Input: part model. Units: mm. Frame: model coordinates. A direction names the side the tool comes from. Round coordinates to 2 decimals unless told otherwise and drop trailing zeros. Loops run counter-clockwise (first coordinate to the right, second up) from the corner with the lowest first, then second, coordinate; pieces in that order, holes last.
1) Ray query, line 1 along X through (y, z) = (74.5, 46.95); line 2 along Z through (x, y) = (170.5, 62); line 3 along Y through (x, z) = (138, 40). Return the intervals inside material, ascending.
2) Section D-D, the plane y = 39. Return loops of the section in (x, z), and give its area (3 significant figures).
3) Section B-B, the plane z = 24.5. Return loops of the section in (x, y).
4) Access query for faces 1 (the face through (201.525, 93, 12)), 2 (the face through (193, 88, 19.5)), 3 (the face through (173.241, 27, 28)), 4 (the face through (180.02, 74.49, 25.08)). Directions: +Z, -Z, +X, -X, +Y, -Y. A direction counts if a zero-diameter tool reaches every point of the face in a straight line with its end or side. Return the directions, or none.
5) Section C-C, the plane x = 63. Return loops of the section in (y, z), and give its area (3 significant figures).
6) Section A-A, the plane z = 41. State how many separate pieces and enclosed holes the cut face has, and give its area (3 significant figures).
7) First-contact query: pin 1 (13.5 mm diameter, centred on x = 112.5, z = 37, fed in from +Y); pin 2 (3 mm diameter, centred on x = 45, z = 9.5, fed in from -Y); pin 3 (12 mm diameter, centred on x = 70, z = 15, fed in from +Y); pin 4 (17.5 mm diameter, centred on x = 121.5, y = 35.5, fed in from +Z). Flat tips, straight axial feed; report the tip coordinate or a pass-through.
8) Draft query along Y for faces 5 (the face through (193, 88, 30.5)), 6 (the face through (48.241, 27, 28)), 7 (the face through (185.44, 94.15, 48.45)). Return one class per face: pulls with the +Y half, pulls with the -Y half, needs draft (parallel to the pull), parting line crosses it, or undercut.
from build123d import *

# Parameters (mm, degrees)
BOSS_EXTRUDE1_DEPTH              = 50
CUT_EXTRUDE1_REACH               = 346.227
CUT_EXTRUDE1_OFFSET_FROM_SURFACE = 10
SKETCH7_W                        = 40
SKETCH7_H                        = 243.120368846
CUT_EXTRUDE2_REACH               = 336.227
SKETCH8_W                        = 40
SKETCH8_H                        = 80.210678119
BOSS_EXTRUDE2_DEPTH              = 5
BOSS_EXTRUDE3_DEPTH              = 5
SKETCH12_W                       = 11
SKETCH12_H                       = 50
CUT_EXTRUDE3_DEPTH               = 20
SKETCH13_W                       = 50
SKETCH13_H                       = 57
BOSS_EXTRUDE4_DEPTH              = 218.275432638
CUT_EXTRUDE5_DEPTH               = 185.855610396
CUT_EXTRUDE5_DEPTH_BACK          = 0.48
SKETCH14_W                       = 40
SKETCH14_H                       = 43.7
SKETCH14_W_2                     = 1.85
CUT_EXTRUDE6_START               = -10
SKETCH15_W                       = 5.5
SKETCH15_H                       = 5
CUT_EXTRUDE6_DEPTH               = 10
SKETCH16_W                       = 125
SKETCH16_H                       = 35
CUT_EXTRUDE7_DEPTH               = 45
CUT_EXTRUDE8_DEPTH               = 5
CUT_EXTRUDE9_DEPTH               = 16.750003
CUT_EXTRUDE10_REACH              = 266.941
SKETCH19_W                       = 6.892135624
SKETCH19_H                       = 14.5
SKETCH20_R                       = 1.75
CUT_EXTRUDE11_DEPTH              = 5


with BuildPart() as part:
    # Sketch2 → Boss-Extrude1 (new body)
    with BuildSketch(Plane.XY):
        Polygon((218.275432638, 103.163478703), (218.275432638, 0), (0, 0), (0, 44.039493547), (0, 248.120368846), (173.241161391, 74.879207455), (201.525432638, 103.163478703), align=None)
    extrude(amount=BOSS_EXTRUDE1_DEPTH)

    # Cut-Extrude1: up to this face of the body (flat: up to its plane, moved by the offset)
    cut_extrude1_end = Plane(part.part.faces().sort_by_distance((86.620580695, 161.499788151, 25))[0]).offset(-CUT_EXTRUDE1_OFFSET_FROM_SURFACE)
    # Sketch7 → Cut-Extrude1 (cut, up to the picked face)
    with BuildSketch(Plane.ZY, mode=Mode.PRIVATE) as cut_extrude1_sk1:
        with Locations((25, 121.560184423)):
            Rectangle(SKETCH7_W, SKETCH7_H)
    cut_extrude1_tool1 = split(extrude(cut_extrude1_sk1.sketch, amount=-CUT_EXTRUDE1_REACH, mode=Mode.PRIVATE), bisect_by=cut_extrude1_end, keep=Keep.BOTH, mode=Mode.PRIVATE)
    add(cut_extrude1_tool1.solids().sort_by(Axis((0, 121.560184, 25), (1, 0, 0)))[0], mode=Mode.SUBTRACT)

    # Cut-Extrude2: up to this plane
    cut_extrude2_end = Plane(origin=(180.312229203, 67.808139643, 50), z_dir=(0.7071067811865477, -0.7071067811865474, 0))
    # Sketch8 → Cut-Extrude2 (cut, up to the surface)
    with BuildSketch(Plane(origin=(218.275432638, 0, 0), x_dir=(0, 0, -1), z_dir=(1, 0, 0)), mode=Mode.PRIVATE) as cut_extrude2_sk1:
        with Locations((-25, 55.808139644)):
            Rectangle(SKETCH8_W, SKETCH8_H)
    cut_extrude2_tool1 = split(extrude(cut_extrude2_sk1.sketch, amount=-CUT_EXTRUDE2_REACH, mode=Mode.PRIVATE), bisect_by=cut_extrude2_end, keep=Keep.BOTH, mode=Mode.PRIVATE)
    add(cut_extrude2_tool1.solids().sort_by_distance((218.275433, 55.80814, 25))[0], mode=Mode.SUBTRACT)

    # Sketch10 → Boss-Extrude2 (add)
    with BuildSketch(Plane.XY.offset(50)):
        Polygon((0, 248.120368846), (3.535533906, 251.655902752), (173.241161391, 81.950275267), (197.989898732, 106.699012609), (201.525432638, 103.163478703), (173.241161391, 74.879207455), align=None)
    extrude(amount=-BOSS_EXTRUDE2_DEPTH)

    # Sketch11 → Boss-Extrude3 (add)
    with BuildSketch(Plane(origin=(0, 0, 0), x_dir=(-1, 0, 0), z_dir=(0, 0, -1))):
        Polygon((-201.525432638, 103.163478703), (-197.989898732, 106.699012609), (-173.241161391, 81.950275267), (-3.535533906, 251.655902752), (0, 248.120368846), (-173.241161391, 74.879207455), align=None)
    extrude(amount=-BOSS_EXTRUDE3_DEPTH)

    # Sketch12 → Cut-Extrude3 (cut)
    with BuildSketch(Plane(origin=(49.180976968, -49.180976968, 0), x_dir=(0, 0, 1), z_dir=(-0.7071067811865435, 0.7071067811865517, 0))):
        with Locations((25, 213.447595361)):
            Rectangle(SKETCH12_W, SKETCH12_H)
    extrude(amount=-CUT_EXTRUDE3_DEPTH, mode=Mode.SUBTRACT)

    # Sketch13 → Boss-Extrude4 (add)
    with BuildSketch(Plane(origin=(218.275432638, 0, 0), x_dir=(0, 0, -1), z_dir=(1, 0, 0))):
        with Locations((-25, 28.5)):
            Rectangle(SKETCH13_W, SKETCH13_H)
    extrude(amount=-BOSS_EXTRUDE4_DEPTH)

    # Sketch14 → Cut-Extrude5 (cut, two sides: drawn at the far end of the back side and taken through both)
    with BuildSketch(Plane(origin=(124.060184423, 124.060184423, 0), x_dir=(0, 0, -1), z_dir=(0.7071067811865435, 0.7071067811865517, 0)).offset(-CUT_EXTRUDE5_DEPTH_BACK)):
        with Locations((-25, -47.702404639)):
            Rectangle(SKETCH14_W, SKETCH14_H)
        with Locations((-45.925, -47.702404639)):
            Rectangle(SKETCH14_W_2, SKETCH14_H)
        with Locations((-4.075, -47.702404639)):
            Rectangle(SKETCH14_W_2, SKETCH14_H)
    extrude(amount=CUT_EXTRUDE5_DEPTH + CUT_EXTRUDE5_DEPTH_BACK, mode=Mode.SUBTRACT)

    # Sketch15 → Cut-Extrude6 (cut)
    with BuildSketch(Plane(origin=(49.180976968, -49.180976968, 0), x_dir=(0, 0, 1), z_dir=(-0.7071067811865477, 0.7071067811865474, 0)).offset(CUT_EXTRUDE6_START)):
        with Locations((27.75, 177.467595361)):
            Rectangle(SKETCH15_W, SKETCH15_H)
        with Locations((22.25, 177.467595361)):
            Rectangle(SKETCH15_W, SKETCH15_H)
    extrude(amount=CUT_EXTRUDE6_DEPTH, mode=Mode.SUBTRACT)

    # Sketch16 → Cut-Extrude7 (cut)
    with BuildSketch(Plane.XY.offset(50)):
        with Locations((110.741161391, 27.5)):
            Rectangle(SKETCH16_W, SKETCH16_H)
    extrude(amount=-CUT_EXTRUDE7_DEPTH, mode=Mode.SUBTRACT)

    # Sketch17 → Cut-Extrude8 (cut)
    with BuildSketch(Plane.XY.offset(5)):
        with BuildLine():
            ThreePointArc((73.991161391, 27.5), (75.741161391, 25.75), (77.491161391, 27.5))
            Line((77.491161391, 27.5), (73.991161391, 27.5))
        make_face()
        with BuildLine():
            Line((73.991161391, 27.5), (77.491161391, 27.5))
            ThreePointArc((77.491161391, 27.5), (75.741161391, 29.25), (73.991161391, 27.5))
        make_face()
        with BuildLine():
            ThreePointArc((108.991161391, 27.5), (110.741161391, 25.75), (112.491161391, 27.5))
            Line((112.491161391, 27.5), (108.991161391, 27.5))
        make_face()
        with BuildLine():
            Line((108.991161391, 27.5), (112.491161391, 27.5))
            ThreePointArc((112.491161391, 27.5), (110.741161391, 29.25), (108.991161391, 27.5))
        make_face()
        with BuildLine():
            ThreePointArc((143.991161391, 27.5), (145.741161391, 25.75), (147.491161391, 27.5))
            Line((147.491161391, 27.5), (143.991161391, 27.5))
        make_face()
        with BuildLine():
            Line((143.991161391, 27.5), (147.491161391, 27.5))
            ThreePointArc((147.491161391, 27.5), (145.741161391, 29.25), (143.991161391, 27.5))
        make_face()
    extrude(amount=-CUT_EXTRUDE8_DEPTH, mode=Mode.SUBTRACT)

    # Sketch18 → Cut-Extrude9 (cut)
    with BuildSketch(Plane(origin=(218.275432638, 0, 0), x_dir=(0, 0, -1), z_dir=(1, 0, 0))):
        Polygon((-5, 95.913478703), (-5, 57), (-45, 57), (-45, 95.913478703), (-30.5, 95.913478703), (-30.5, 103.163478703), (-50, 103.163478703), (-50, 0), (0, 0), (0, 103.163478703), (-19.5, 103.163478703), (-19.5, 95.913478703), align=None)
    extrude(amount=-CUT_EXTRUDE9_DEPTH, mode=Mode.SUBTRACT)

    # Sketch19 → Cut-Extrude10 (cut, up to next)
    with BuildSketch(Plane(origin=(0, 95.913478703, 0), x_dir=(1, 0, 0), z_dir=(0, 1, 0)), mode=Mode.PRIVATE) as cut_extrude10_sk1:
        with Locations((204.97150045, -37.75)):
            Rectangle(SKETCH19_W, SKETCH19_H)
    cut_extrude10_tool1 = extrude(cut_extrude10_sk1.sketch, amount=-CUT_EXTRUDE10_REACH, mode=Mode.PRIVATE) & part.part
    # Sketch19 → Cut-Extrude10 (cut, up to next)
    with BuildSketch(Plane(origin=(0, 95.913478703, 0), x_dir=(1, 0, 0), z_dir=(0, 1, 0)), mode=Mode.PRIVATE) as cut_extrude10_sk2:
        with Locations((204.97150045, -12.25)):
            Rectangle(SKETCH19_W, SKETCH19_H)
    cut_extrude10_tool2 = extrude(cut_extrude10_sk2.sketch, amount=-CUT_EXTRUDE10_REACH, mode=Mode.PRIVATE) & part.part
    add(cut_extrude10_tool1.solids().sort_by_distance((204.9715, 95.913479, 37.75))[0], mode=Mode.SUBTRACT)
    add(cut_extrude10_tool2.solids().sort_by_distance((204.9715, 95.913479, 12.25))[0], mode=Mode.SUBTRACT)

    # Sketch20 → Cut-Extrude11 (cut)
    with BuildSketch(Plane.XY.offset(50)):
        with Locations((176.525432638, 74.5)):
            Circle(SKETCH20_R)
        with Locations((160.025432638, 74.5)):
            Circle(SKETCH20_R)
        with Locations((193.025432638, 74.5)):
            Circle(SKETCH20_R)
    extrude(amount=-CUT_EXTRUDE11_DEPTH, mode=Mode.SUBTRACT)


solid = part.part
Final values:
1. line 1: x = 0 to 158.28, 161.78 to 174.78, 178.28 to 191.28, 194.78 to 201.53
1. line 2: z = 0 to 5, 45 to 50
1. line 3: y = 0 to 10, 45 to 57, 95.98 to 110.12
2. outline: (0, 0) - (201.53, 0) - (201.53, 50) - (173.24, 50) - (173.24, 5) - (48.24, 5) - (48.24, 50) - (0, 50) - close
2. area: 4,450 mm2
3. outline: (0, 0) - (201.53, 0) - (201.53, 57) - (0, 57) - close; (0, 233.98) - (173.24, 60.74) - (179.97, 67.47) - (142, 105.44) - (142.34, 105.78) - (0, 248.12) - close; (176.44, 78.08) - (183.51, 71) - (189.5, 77) - (182.43, 84.07) - close; hole (48.24, 10) - (173.24, 10) - (173.24, 45) - (48.24, 45) - close
4. face 1: +Z, -Z, +X, +Y, -Y
4. face 2: +X, +Y
4. face 3: +Z
4. face 4: none
5. outline: (0, 0) - (192.19, 0) - (192.19, 5) - (185.12, 5) - (185.12, 45) - (192.19, 45) - (192.19, 50) - (45, 50) - (45, 5) - (10, 5) - (10, 50) - (0, 50) - close; hole (57, 5) - (170.98, 5) - (170.98, 45) - (57, 45) - close
5. area: 3,190 mm2
6. separate pieces: 2
6. enclosed holes: 1
6. area: 9,940 mm2
7. pin 1: stops at y = 142.37
7. pin 2: stops at y = 0
7. pin 3: stops at y = 184.12
7. pin 4: stops at z = 5
8. face 5: needs draft
8. face 6: undercut
8. face 7: pulls with the +Y half
